For this review, take the finished solid that the model builds, in its own axes (mm). A direction names the side the tool comes from. Give positions to 0.01 mm unless a question says otherwise; leave off trailing zeros. Write each loop counter-clockwise with the first axis right and the second up, starting at its lowest first coordinate (ties: lowest second). Pieces come first, ordered by that corner, then holes.
1) For P1, Ø8, axis at x = -24.5, z = 46, coming from the -Y side; P2, Ø9, axis at x = -8.5, y = 29, coming from the -Z side, all flat-tipped, find the tip position at first contact; note any pin that passes through.
2) Machinability: for faces 1 (the face through (1, 30, 50.5)), 2 (the face through (-40, 54, 41)), which of the approach directions +Z, -Z, +X, -X, +Y, -Y give a long, thin tool a straight path to every point of the face, cutting with its end or side? Answer none if there is none.
3) We need section A-A on x = -21. Give the boundary of the cut face in (y, z).
4) We need section B-B on z = -37.5. Give the boundary of the cut face in (x, y), and give its area (3 significant figures).
5) Wall thickness on line 1 along Y through (x, z) = (-15.5, 7); line 2 along Z through (x, y) = (14, 37.5): over which ranges is each line inside the solid? List them lowest first.
6) We need section C-C on y = 19. Give the boundary of the cut face in (x, z), and give its area (3 significant figures).
from build123d import *

# Parameters (mm, degrees)
SKETCH003_W     = 150
SKETCH003_H     = 80
PAD001_DEPTH    = 65
SKETCH004_W     = 100.5
SKETCH004_H     = 60
POCKET002_DEPTH = 30
SKETCH005_W     = 30
SKETCH005_H     = 100.5
POCKET003_DEPTH = 80.001


with BuildPart() as part:
    # Sketch003 (on Face1 of CopyChamfer002) → Pad001 (new body)
    with BuildSketch(Plane.ZX.offset(15)):
        with Locations((25, 0)):
            Rectangle(SKETCH003_W, SKETCH003_H)
    extrude(amount=PAD001_DEPTH)

    # Sketch004 (on Face5 of Pad001) → Pocket002 (cut)
    with BuildSketch(Plane(origin=(0, 15, 0), x_dir=(0, 0, -1), z_dir=(0, -1, 0))):
        with Locations((-0.25, 0)):
            Rectangle(SKETCH004_W, SKETCH004_H)
    extrude(amount=-POCKET002_DEPTH, mode=Mode.SUBTRACT)

    # Sketch005 (on Face1 of Pocket002) → Pocket003 (cut, through all)
    with BuildSketch(Plane.YZ.offset(40)):
        with Locations((30, 0.25)):
            Rectangle(SKETCH005_W, SKETCH005_H)
    extrude(amount=-POCKET003_DEPTH, mode=Mode.SUBTRACT)


solid = part.part
Results list:
1. P1: stops at y = 45
1. P2: stops at z = 50.5
2. face 1: -Z, +X, -X, -Y
2. face 2: +Z, -Z, -X, +Y, -Y
3. outline: (15, 50.5) - (45, 50.5) - (45, -50) - (80, -50) - (80, 100) - (15, 100) - close
4. outline: (-40, 45) - (40, 45) - (40, 80) - (-40, 80) - close
4. area: 2,800 mm2
5. line 1: y = 45 to 80
5. line 2: z = 50.5 to 100
6. outline: (-40, 50.5) - (40, 50.5) - (40, 100) - (-40, 100) - close
6. area: 3,960 mm2
